Autodesk Inventor part; units mm, degrees
ref_plane "YZ Plane" through (0, 0, 0) normal (1, 0, 0) x (0, 1, 0)
ref_plane "XZ Plane" through (0, 0, 0) normal (0, 1, 0) x (-1, 0, 0)
ref_plane "XY Plane" through (0, 0, 0) normal (0, 0, 1) x (1, 0, 0)
sketch "Sketch1" plane through (0, 0, 0) normal (0, 0, 1) x (1, 0, 0)
  line L0 (5, 82.875) -> (-5, 82.875)
  line L1 (-5, 82.875) -> (-5, -82.875)
  line L2 (-5, -82.875) -> (5, -82.875)
  line L3 (5, -82.875) -> (5, 82.875)
  line L4 (-2.05, 24.575) -> (2.05, 24.575)
  line L5 (2.05, 24.575) -> (2.05, 28.675)
  line L6 (2.05, 28.675) -> (-2.05, 28.675)
  line L7 (-2.05, 28.675) -> (-2.05, 24.575)
  line L8 (-2.05, -24.575) -> (2.05, -24.575)
  line L9 (2.05, -24.575) -> (2.05, -28.675)
  line L10 (2.05, -28.675) -> (-2.05, -28.675)
  line L11 (-2.05, -28.675) -> (-2.05, -24.575)
  line L12 (0, -28.675) -> (0, 28.675)
  line L13 (-5, 0) -> (0, 0)
  line L14 (-2.05, 82.875) -> (-2.05, 79.875)
  line L15 (-2.05, 79.875) -> (-5, 79.875)
  line L16 (2.05, 82.875) -> (2.05, 79.875)
  line L17 (2.05, 79.875) -> (5, 79.875)
  line L18 (-2.05, -82.875) -> (-2.05, -79.875)
  line L19 (-2.05, -79.875) -> (-5, -79.875)
  line L20 (2.05, -82.875) -> (2.05, -79.875)
  line L21 (2.05, -79.875) -> (5, -79.875)
  line L22 (5, -79.875) -> (10, -79.875)
  line L23 (-5, -79.875) -> (-10, -79.875)
  line L24 (5, 79.875) -> (10, 79.875)
  line L25 (-5, 79.875) -> (-10, 79.875)
  arc A0 (10, 79.875) -> (10, -79.875) centre (645.5016, 0) ccw
  arc A1 (-10, -79.875) -> (-10, 79.875) centre (-645.5016, 0) ccw
  point P0 (5, 0)
  dimension "d0" = 10
  dimension "d1" = 165.75
  dimension "d4" = 4.1
  dimension "d5" = 4.1
  dimension "d6" = 49.15
  dimension "d7" = 4.1
  dimension "d8" = 4.1
  dimension "d9" = 5
  dimension "d10" = 3
  dimension "d11" = 3
  dimension "d18" = 5
  dimension "d19" = 5
  dimension "d20" = 5
  dimension "d21" = 5
extrude "Extrusion1" add sketch "Sketch1" along normal blind 4 contours L16 L17 L3 L21 L20 L2 L18 L19 L1 L15 L14 L0 | L24 A0 L3 | A0 L22 L3 | L1 A1 L25 | L1 L23 A1
chamfer "Chamfer1" distance 0.5 angle 45 12 edges at (0, 82.875, 4) (-2.05, 82.875, 2) (0, 82.875, 0) (2.05, 82.875, 2) (2.05, -82.875, 2) (0, -82.875, 4) (-2.05, -82.875, 2) (0, -82.875, 0) (2.05, 26.625, 0) (-2.05, 26.625, 0) (2.05, -26.625, 0) (-2.05, -26.625, 0)
chamfer "Chamfer2" distance 0.75 angle 45 4 edges at (0, 28.675, 0) (0, 24.575, 0) (0, -24.575, 0) (0, -28.675, 0)
equation "\"d5\" = d4"
equation "\"d7\" = d4"
equation "\"d8\" = d4"
equation "\"d9\" = 0.5 * d0"
equation "\"d19\" = d18"
equation "\"d20\" = d18"
equation "\"d21\" = d18"
properties part number "BareCalibrationClipSide"
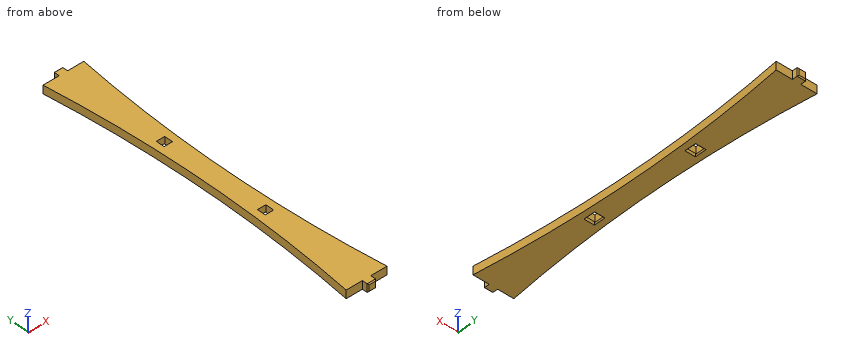
Build history of the part. All positions in model axes, mm. Coordinates: 2 decimals unless noted, no trailing zeros. Write each loop counter-clockwise with the first axis right and the second up, starting at its lowest first coordinate (ties: lowest second). Pieces come first, ordered by that corner, then holes.
1. Band-saw the part on D-D, the plane y = -44.5. Give the cut face in (x, z).
Answer block:
outline: (-6.55, 0) - (6.55, 0) - (6.55, 4) - (-6.55, 4) - close
2. Drop flat-ended pins along their axis: pin 1 (2 mm diameter, centred on y = -32.5, z = 2.5, fed in from +X); pin 2 (2 mm diameter, centred on x = -4, z = 1, fed in from -Y) (3 decimals); pin 3 (2 mm diameter, centred on y = -81, z = 1.5, fed in from -X). Give the stop position or say it passes through.
Answer block:
pin 1: stops at x = 5.88
pin 2: stops at y = -79.875
pin 3: stops at x = -2.05
3. Band-saw the part on B-B, the plane x = -8.25. Give the cut face in (y, z) (3 decimals), and give its area (3 significant figures).
Answer block:
outline: (-79.875, 0) - (-64.441, 0) - (-64.441, 4) - (-79.875, 4) - close; (64.441, 0) - (79.875, 0) - (79.875, 4) - (64.441, 4) - close
area: 123 mm2
4. Band-saw the part on C-C, the plane y = -12.5. Give the cut face in (x, z).
Answer block:
outline: (-5.12, 0) - (5.12, 0) - (5.12, 4) - (-5.12, 4) - close
5. Drill centre lines: probe 1 along Y at (x, z) = (-1, 1.05) (3 decimals); probe 2 along Y at (x, z) = (-1.75, 1.9) (3 decimals); probe 3 along Y at (x, z) = (3.5, 0.3) (3 decimals). Where is each one in solid material? Low to high.
Answer block:
probe 1: y = -82.875 to -28.675, -24.575 to 24.575, 28.675 to 82.875
probe 2: y = -82.675 to -28.675, -24.575 to 24.575, 28.675 to 82.675
probe 3: y = -79.875 to 79.875
6. Band-saw the part on A-A, the plane z = 2.3. Give the cut face in (x, y) (3 decimals).
Answer block:
outline: (-10, -79.875) - (-2.05, -79.875) - (-2.05, -82.375) - (-1.55, -82.875) - (1.55, -82.875) - (2.05, -82.375) - (2.05, -79.875) - (10, -79.875) arc R640.502 cw to (10, 79.875) - (2.05, 79.875) - (2.05, 82.375) - (1.55, 82.875) - (-1.55, 82.875) - (-2.05, 82.375) - (-2.05, 79.875) - (-10, 79.875) arc R640.502 cw to start; hole (-2.05, -28.675) - (2.05, -28.675) - (2.05, -24.575) - (-2.05, -24.575) - close; hole (-2.05, 24.575) - (2.05, 24.575) - (2.05, 28.675) - (-2.05, 28.675) - close
